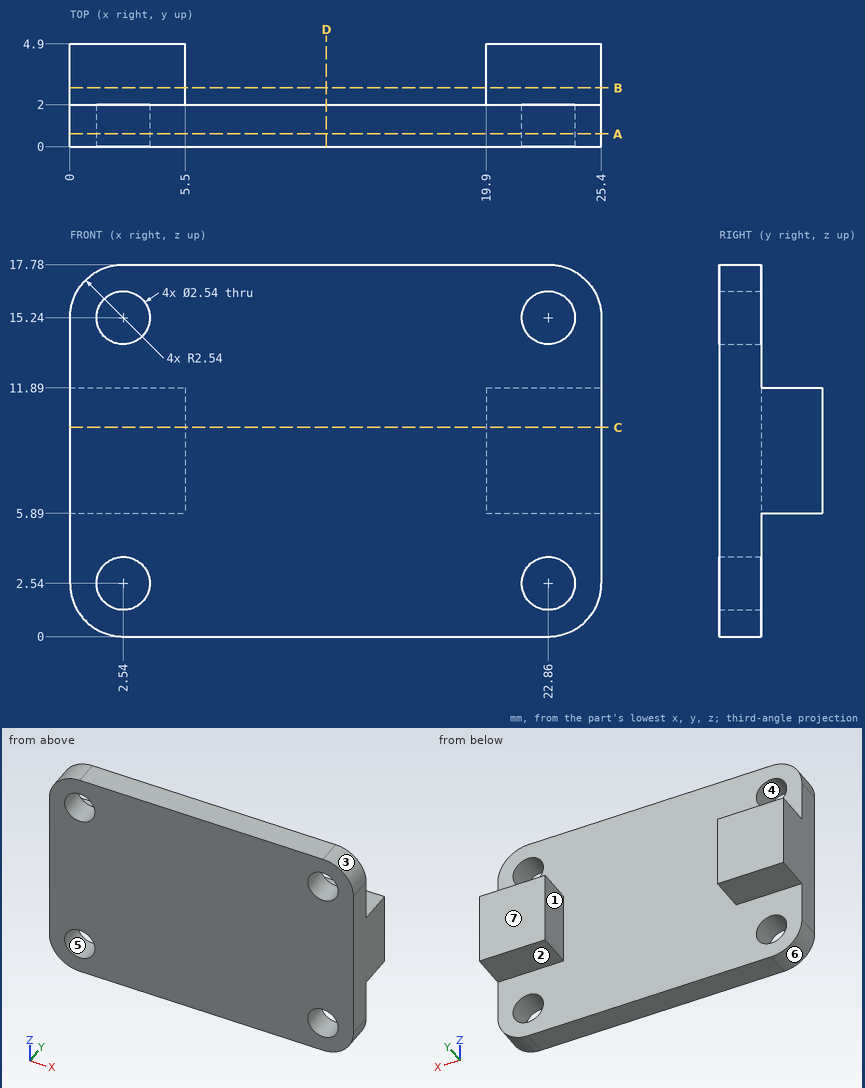
Here's the drawing with two shaded views (mm, measured from the low corner). I have some questions. A direction names the side the tool comes from. Coordinates: 2 decimals unless noted, no trailing zeros. Loops run counter-clockwise (first coordinate to the right, second up) from the corner with the lowest first, then second, coordinate; pieces in that order, holes last. Notation, with made-up numbers: M 81,-6.5 L 119,-6.5 A36 cw 119,32.5 Z; hole C 81,-30 d3. An arc over 180 degrees is marked long. Return JSON: item names as keys, results as strings. Group by question number.
Item 1: On a 3-axis mill with a long thin cutter (end or side, diameter ignored), from which of +Z, -Z, +X, -X, +Y, -Y can I reach the whole of each face in a straight line? I mean the marked faces 1, 2 and 3. Say none if no direction works.
Item 2: If I drill on L1, parallel to Z at x = 22.86, y = 0.8; L2, parallel to X at y = 3.75, z = 8.25; L3, parallel to X at y = 1.05, z = 1.5, over which ranges is the centre line in solid material (lowest first)? Write a range as from..to.
Item 3: Imagine slicing it at A-A (y = 0.6). Please give me the cut outline in (x, z).
Item 4: I'm going to push flat-ended pins straight in: pin 1 Ø3.5 at (x, z) = (22.86, 2.54) entering from +Y; pin 2 Ø1.5 at (x, y) = (2.5, 4) entering from -Z; pin 3 Ø0.9 at (x, y) = (3, 3) entering from +Z. Where does each tip first touch, or does it pass through?
Item 5: Thinking about a two-plate mould opening in X: for the marked faces 4, 5, 6 and 7, which applies, released by +X, released by -X, zero draft, split by the parting line, or undercut?
Item 6: Imagine slicing it at D-D (x = 12.25). Please give me the cut outline in (y, z), and give its area (3 significant figures).
Item 7: Imagine slicing it at C-C (z = 10). Please give me the cut outline in (x, y).
Item 8: Imagine slicing it at B-B (y = 2.8). Please give me the cut outline in (x, z).
Verdict:
{
 "1": {"face 1": "+Z, -Z, +Y", "face 2": "-Z, +X, -X, +Y", "face 3": "+Z, +X, +Y, -Y"},
 "2": {"L1": "z = 0..1.27, 3.81..13.97, 16.51..17.78", "L2": "x = 0..5.5, 19.9..25.4", "L3": "x = 0.22..1.81, 3.27..22.13, 23.59..25.18"},
 "3": {"outline": "M 0,2.54 A2.54 ccw 2.54,0 L 22.86,0 A2.54 ccw 25.4,2.54 L 25.4,15.24 A2.54 ccw 22.86,17.78 L 2.54,17.78 A2.54 ccw 0,15.24 Z; hole C 2.54,2.54 d2.54; hole C 2.54,15.24 d2.54; hole C 22.86,2.54 d2.54; hole C 22.86,15.24 d2.54"},
 "4": {"pin 1": "stops at y = 2", "pin 2": "stops at z = 5.89", "pin 3": "stops at z = 11.89"},
 "5": {"face 4": "undercut", "face 5": "undercut", "face 6": "released by -X", "face 7": "zero draft"},
 "6": {"outline": "M 0,0 L 2,0 L 2,17.78 L 0,17.78 Z", "area": "35.6 mm^2"},
 "7": {"outline": "M 0,0 L 25.4,0 L 25.4,4.9 L 19.9,4.9 L 19.9,2 L 5.5,2 L 5.5,4.9 L 0,4.9 Z"},
 "8": {"outline": "M 0,5.89 L 5.5,5.89 L 5.5,11.89 L 0,11.89 Z; M 19.9,5.89 L 25.4,5.89 L 25.4,11.89 L 19.9,11.89 Z"}
}
